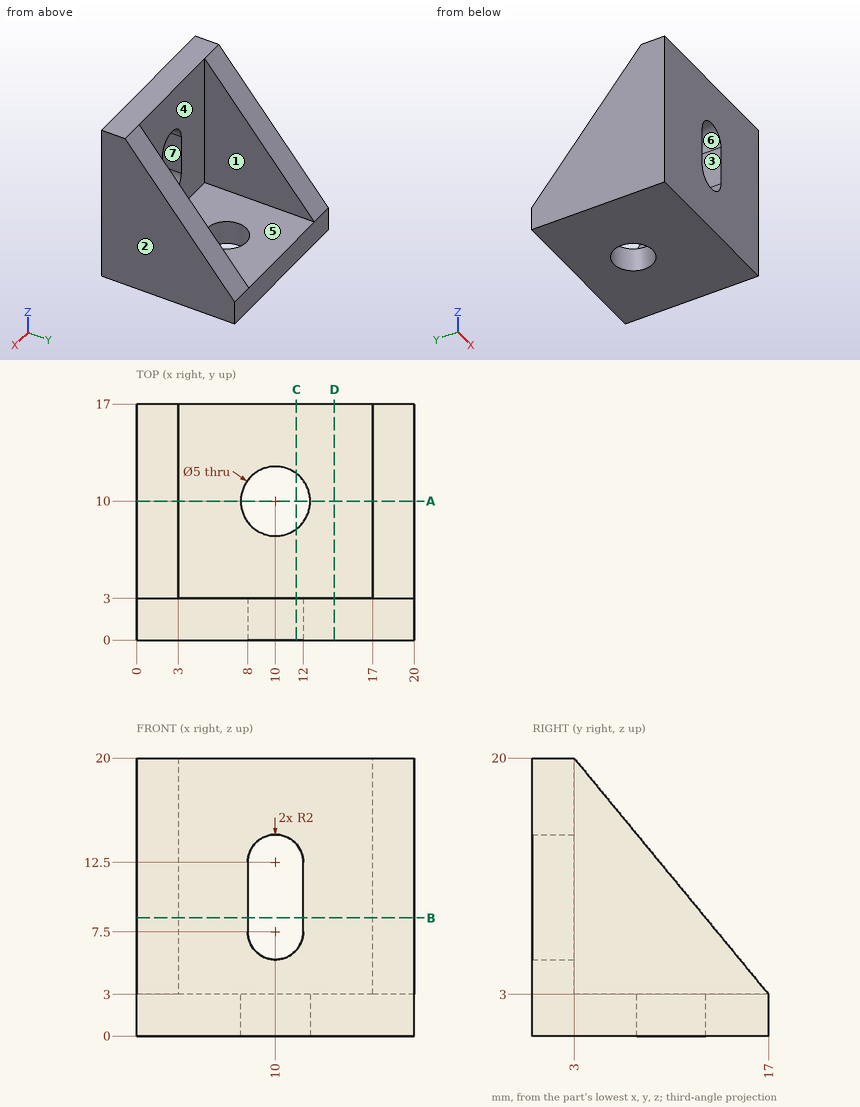
Geometry check sheet. Reference: drawing and pictorial views, mm from the part's lowest x, y, z. A direction names the side the tool comes from. Coordinates: 2 decimals unless noted, no trailing zeros. Write each loop counter-clockwise with the first axis right and the second up, starting at its lowest first coordinate (ties: lowest second). Pieces come first, ordered by that corner, then holes. Notation, with made-up numbers: (-8, -1) - (51, -1) arc R32 ccw to (51, 33) - close; hole circle Ø11 at (-36.5, 15.25). An arc over 180 degrees is marked (long way). Write item = value, one per line.
Q1. Cross-section at D-D (x = 14.25). Enter the section's corners in (y, z), plus the area to 3 significant figures.
Answer:
outline = (0, 0) - (17, 0) - (17, 3) - (3, 3) - (3, 20) - (0, 20) - close
area = 102 mm²
Q2. Go/stop test with flat-tipped pins: pin 1 Ø2 at (x, z) = (11.5, 16) entering from -Y; pin 2 Ø4 at (x, y) = (7, 10.5) entering from +Z; pin 3 Ø7 at (x, z) = (7, 10.5) entering from +Y. Record where each tip stops, or that it passes through.
Answer:
pin_1 = 0
pin_2 = 3
pin_3 = 3
Q3. Mould release check, pull along Z, two halves, no side actions. Record for the marked faces 4, 5, 6 and 7: released by +Z, released by -Z, zero draft, split by the parting line, or undercut.
Answer:
face_4 = zero draft
face_5 = released by +Z
face_6 = undercut
face_7 = undercut
Q4. Access from +Z, -Z, +X, -X, +Y, -Y to the whole of each face (thin tool, end or side, straight path). Record for the marked faces 1, 2 and 3.
Answer:
face_1 = +Z, +Y
face_2 = +Z, -Z, +X, +Y, -Y
face_3 = +Y, -Y
Q5. Cross-section at C-C (x = 11.5). Enter the section's corners in (y, z), plus the area to 3 significant figures.
Answer:
outline = (0, 0) - (8, 0) - (8, 3) - (3, 3) - (3, 6.18) - (0, 6.18) - close; (0, 13.82) - (3, 13.82) - (3, 20) - (0, 20) - close; (12, 0) - (17, 0) - (17, 3) - (12, 3) - close
area = 67.1 mm²
Q6. Cross-section at A-A (y = 10). Enter the section's corners in (x, z).
Answer:
outline = (0, 0) - (7.5, 0) - (7.5, 3) - (3, 3) - (3, 11.5) - (0, 11.5) - close; (12.5, 0) - (20, 0) - (20, 11.5) - (17, 11.5) - (17, 3) - (12.5, 3) - close
Q7. Material ranges on L1, parallel to Y at x = 10, z = 2.35; L2, parallel to X at y = 4.25, z = 11.25; L3, parallel to Z at x = 6.75, y = 15, recorded low to high. Write a range as from..to.
Answer:
L1 = 0..7.5, 12.5..17
L2 = 0..3, 17..20
L3 = 0..3
Q8. Cross-section at B-B (z = 8.5). Enter the section's corners in (x, y), plus the area to 3 significant figures.
Answer:
outline = (0, 0) - (8, 0) - (8, 3) - (3, 3) - (3, 12.47) - (0, 12.47) - close; (12, 0) - (20, 0) - (20, 12.47) - (17, 12.47) - (17, 3) - (12, 3) - close
area = 105 mm²
